Design review of the part built by this model. Coordinates are the model's own, in mm. A direction names the side the tool comes from. Give positions to 0.01 mm unless a question says otherwise; leave off trailing zeros. Write each loop counter-clockwise with the first axis right and the second up, starting at its lowest first coordinate (ties: lowest second). Pieces come first, ordered by that corner, then holes. Notation, with made-up numbers: (85.25, 4.5) -> (124.25, 4.5) arc R16 ccw to (124.25, 15.5) -> close; hole circle Ø1 at (81.25, -29.5). An arc over 180 degrees is marked (long way). Use CSV: the item, a comma, the result in double quotes.
```python
from build123d import *

# Parameters (mm, degrees)
SKETCH1_W           = 3
SKETCH1_H           = 15
SKETCH1_W_2         = 12.413793103
SKETCH1_H_2         = 3
BOSS_EXTRUDE1_DEPTH = 16
SKETCH2_W           = 34
SKETCH2_H           = 18
BOSS_EXTRUDE2_DEPTH = 3


with BuildPart() as part:
    # Sketch1 → Boss-Extrude1 (new body)
    with BuildSketch(Plane(origin=(0, 0, 0), x_dir=(1, 0, 0), z_dir=(0, 1, 0))):
        with Locations((-18.5, -2.557471264)):
            Rectangle(SKETCH1_W, SKETCH1_H)
        with Locations((-23.206896552, -11.557471264)):
            Rectangle(SKETCH1_W_2, SKETCH1_H_2)
        Polygon((0, 7.942528736), (-20, 7.942528736), (-20, 4.942528736), (-17, 4.942528736), (0, 4.942528736), align=None)
        Polygon((20, 7.942528736), (0, 7.942528736), (0, 4.942528736), (17, 4.942528736), (20, 4.942528736), align=None)
        with Locations((18.5, -2.557471264)):
            Rectangle(SKETCH1_W, SKETCH1_H)
        Polygon((29.413793103, -10.057471264), (20, -10.057471264), (17, -10.057471264), (17, -13.057471264), (29.413793103, -13.057471264), align=None)
    extrude(amount=BOSS_EXTRUDE1_DEPTH)

    # Sketch2 → Boss-Extrude2 (add)
    with BuildSketch(Plane(origin=(0, 0, 0), x_dir=(1, 0, 0), z_dir=(0, 1, 0))):
        with Locations((0, -4.057471264)):
            Rectangle(SKETCH2_W, SKETCH2_H)
    extrude(amount=BOSS_EXTRUDE2_DEPTH)


solid = part.part
```
(1) Clearance check with flat-ended pins moving along their axes: pin 1 (7.5 mm diameter, centred on x = -26, y = 7, fed in from -Z); pin 2 (4 mm diameter, centred on x = 7.5, y = 11, fed in from +Z); pin 3 (6.5 mm diameter, centred on y = 8, z = 3.5, fed in from -X); pin 4 (3 mm diameter, centred on x = 0.5, z = 7, fed in from -Y). State where each tip first meets the part, or that it passes through.
Established:
pin 1,"stops at z = 10.06"
pin 2,"stops at z = -4.94"
pin 3,"stops at x = -20"
pin 4,"stops at y = 0"
(2) Take a section at B-B (y = 11). Write out the cut boundary in (x, z), then the cut area to 3 significant figures.
Established:
outline,"(-29.41, 10.06) -> (-20, 10.06) -> (-20, -7.94) -> (20, -7.94) -> (20, 10.06) -> (29.41, 10.06) -> (29.41, 13.06) -> (17, 13.06) -> (17, -4.94) -> (-17, -4.94) -> (-17, 13.06) -> (-29.41, 13.06) -> close"
area,"284 mm2"
(3) Take a section at D-D (z = 11.75). Write out the cut boundary in (x, y).
Established:
outline,"(-29.41, 0) -> (29.41, 0) -> (29.41, 16) -> (17, 16) -> (17, 3) -> (-17, 3) -> (-17, 16) -> (-29.41, 16) -> close"
(4) For line 1 along X through (y, z) = (7, 11.25); line 2 along X through (y, z) = (7, 7.25); line 3 along Z through (x, y) = (3, 11), list the stretches that pass through material, from the lowest coordinate up. Write a range as [from, to].
Established:
line 1,"x = [-29.41, -17], [17, 29.41]"
line 2,"x = [-20, -17], [17, 20]"
line 3,"z = [-7.94, -4.94]"
(5) Take a section at C-C (x = -25). Write out the cut boundary in (y, z), then the cut area to 3 significant figures.
Established:
outline,"(0, 10.06) -> (16, 10.06) -> (16, 13.06) -> (0, 13.06) -> close"
area,"48.0 mm2"
(6) Take a section at A-A (z = 5.75). Write out the cut boundary in (x, y), then the cut area to 3 significant figures.
Established:
outline,"(-20, 0) -> (20, 0) -> (20, 16) -> (17, 16) -> (17, 3) -> (-17, 3) -> (-17, 16) -> (-20, 16) -> close"
area,"198 mm2"
(7) Mouldability with a two-part tool opening along X and no side actions: class faces 4 (the face through (0, 9, -4.943)), 5 (the face through (-25, 8, 10.057)), 6 (the face through (-20, 8, 1)), 7 (the face through (29.414, 8, 12)) as +X half, -X half, draft (parallel to the pull), parting line (faces both ways), or undercut.
Established:
face 4,"undercut"
face 5,"draft"
face 6,"-X half"
face 7,"+X half"
(8) Tool access review of faces 1 (the face through (-29.414, 8, 12)), 2 (the face through (25, 8, 10.057)), 3 (the face through (0, 3, 4)): name each direction out of +Z, -Z, +X, -X, +Y, -Y from which nothing blocks a thin tool from reaching the whole face with its end or side.
Established:
face 1,"+Z, -Z, -X, +Y, -Y"
face 2,"-Z, +X, +Y, -Y"
face 3,"+Z, +Y"
